Check sheet for the modelled part. Datum: model origin and axes. Units: mm. Round coordinates to 2 decimals unless told otherwise and drop trailing zeros. Order: outer loops, then holes, each group sorted by start corner. A loop starts at its lowest first (then second) coordinate and runs counter-clockwise, first axis right, second up.
Q1. Cross-section at B-B on y = 135.5. Record the cut outline in (x, z), then the cut area to 3 significant figures.
Q2. Scan lines: probe 1 along X at (y, z) = (127, -1); probe 2 along Y at (x, z) = (5, -31); probe 3 along Z at (x, y) = (0, 674). Record each from-to range of solid material in increasing order.
Q3. Cross-section at A-A on z = 0. Record the cut outline in (x, y).
Q4. Mould release check, pull along X, two halves, no side actions. Record for faces 1 (the flat face through (17, 1270, -19.4)), 2 (the cylindrical face through (-30.235, 626.181, -23.183)), 3 (the cylindrical face through (-5.506, 626.11, -24.796)): +X half, -X half, draft (parallel to the pull), parting line (faces both ways), or undercut.
Q5. Depth check by flat-ended pin: P1, Ø13, axis at x = 0, y = 177.8, coming from the +Z side; P2, Ø1.5, axis at y = 992, z = 18, coming from the +X side; P3, Ø1.5, axis at y = 164, z = -21, coming from the +X side; P4, Ø5, axis at x = -16.5, y = 1075.5, coming from the +Z side. Enter the tip coordinate at first touch or a pass-through.
from build123d import *

# Parameters (mm, degrees)
F0_R     = 38.1
F1_DEPTH = 1270
F2_R     = 25.4
F3_DEPTH = 1270.001
F4_R     = 5.08
F6_DEPTH = 38.1


with BuildPart() as f1:
    # F0 (on Front) → F1 (new body)
    with BuildSketch(Plane.XZ):
        Circle(F0_R)
    extrude(amount=-F1_DEPTH)

    # F2 (on face) → F3 (cut, through all)
    with BuildSketch(Plane.XZ):
        Circle(F2_R)
    extrude(amount=-F3_DEPTH, mode=Mode.SUBTRACT)

    # F4
    f4_edges = [f1.edges().sort_by_distance(p)[0] for p in [
        (-38.1, 0, 0),
        (-38.1, 1270, 0),
    ]]
    fillet(f4_edges, radius=F4_R)

    # F5 (on Top) → F6 (cut, symmetric)
    with BuildSketch(Plane.XY):
        with BuildLine():
            ThreePointArc((0, 172.085), (4.041115, 173.758885), (5.715, 177.8))
            ThreePointArc((5.715, 177.8), (-4.041115, 181.841115), (0, 172.085))
        make_face()
        with BuildLine():
            ThreePointArc((5.715, 25.4), (4.041115, 29.441115), (0, 31.115))
            ThreePointArc((0, 31.115), (-5.715, 25.4), (0, 19.685))
            ThreePointArc((0, 19.685), (4.041115, 21.358885), (5.715, 25.4))
        make_face()
    extrude(amount=F6_DEPTH, both=True, mode=Mode.SUBTRACT)


solid = f1.part
Results found:
1. outline: circle Ø76.2 at (0, 0); hole circle Ø50.8 at (0, 0)
1. area: 2,530 mm2
2. probe 1: x = -38.09 to -25.38, 25.38 to 38.09
2. probe 2: y = 0 to 22.63, 28.17 to 175.03, 180.57 to 1270
2. probe 3: z = -38.1 to -25.4, 25.4 to 38.1
3. outline: (-38.1, 5.08) arc R5.08 ccw to (-33.02, 0) - (-25.4, 0) - (-25.4, 1270) - (-33.02, 1270) arc R5.08 ccw to (-38.1, 1264.92) - close; (25.4, 0) - (33.02, 0) arc R5.08 ccw to (38.1, 5.08) - (38.1, 1264.92) arc R5.08 ccw to (33.02, 1270) - (25.4, 1270) - close
4. face 1: draft
4. face 2: parting line
4. face 3: undercut
5. P1: stops at z = 38.1
5. P2: stops at x = 33.97
5. P3: stops at x = 32.27
5. P4: stops at z = 35.43
